The listing builds one solid part. Answer for the finished solid, in the listing's coordinates (mm). A direction names the side the tool comes from. Round coordinates to 2 decimals unless told otherwise and drop trailing zeros. Loops run counter-clockwise (first coordinate to the right, second up) from the corner with the lowest first, then second, coordinate; pieces in that order, holes last. Notation, with made-up numbers: M -33.75,24 L 24.25,24 A21 cw 24.25,36 Z; hole C -18,-35 d5. An arc over 180 degrees is marked long. Put each result on its own line as item: value. Start each with the question number.
(1) Determine the mould class of faces 4 (the face through (54, -2, -72)), 5 (the face through (34.359, -1.726, 79.113)), 6 (the face through (42.922, -1.726, -52.965)) for opening direction Z: released by +Z, released by -Z, zero draft, split by the parting line, or undercut.
(2) Straight lines are drawn through the part: line 1 (Z direction, x = 46, y = -2.2); line 2 (Z direction, x = 73.5, y = -1.1); line 3 (X direction, y = -2.25, z = -44). For each, find the intervals that lie inside material, in ascending order.
(3) Section B-B, the plane y = -2.25 is taken. Count the separate pieces of the cut face and the enclosed holes in it, then the cut area to 3 significant figures.
(4) Section D-D, the plane z = -35 is taken. Determine the outline of the cut face in (x, y), then the cut area to 3 significant figures.
(5) Section C-C, the plane z = 3 is taken. Determine the outline of the cut face in (x, y), then the cut area to 3 significant figures.
(6) Which of the six approach directions +Z, -Z, +X, -X, +Y, -Y give full straight-line access (tool end or side, diameter ignored) to faces 1 (the face through (50.873, -2, -47)), 2 (the face through (60.112, -1.726, 66.981)), 3 (the face through (59.328, -1.726, -3.284))?
(7) Flat-ended cylindrical pins translate along their axes: P1, Ø0.7, axis at y = -2.5, z = -43, coming from the -X side; P2, Ø2, axis at x = 77.5, y = -2, coming from the +Z side; P3, Ø1, axis at y = -1.5, z = -48, coming from the -X side. Find the tip coordinate at first contact, or state that the pin passes through.
(8) Section A-A, the plane x = 45 is taken. Determine the outline of the cut face in (y, z), then the cut area to 3 significant figures.
```python
from build123d import *

# Parameters (mm, degrees)
F1_DEPTH = 3.5
F2_D     = 7.5
F4_DEPTH = 25


with BuildPart() as f1:
    # F0 (on Front) → F1 (new body)
    with BuildSketch(Plane.XZ):
        with BuildLine():
            ThreePointArc((41.4336819508, -79.5), (42.1706374775, -79.4080743718), (42.8624296043, -79.1379310345))
            ThreePointArc((42.8624296043, -79.1379310345), (90, 0), (42.8624296043, 79.1379310345))
            ThreePointArc((42.8624296043, 79.1379310345), (42.1706374775, 79.4080743718), (41.4336819508, 79.5))
            Line((41.4336819508, 79.5), (35.8331652233, 79.5))
            ThreePointArc((35.8331652233, 79.5), (34.3404775581, 79.1022842916), (33.2435667811, 78.0145890229))
            ThreePointArc((33.2435667811, 78.0145890229), (30.1884169541, 62.5971202701), (37.3284684526, 48.5952651142))
            ThreePointArc((37.3284684526, 48.5952651142), (37.696787223, 48.2936203298), (38.1081859652, 48.054038679))
            ThreePointArc((38.1081859652, 48.054038679), (53.4450002112, 35.0932650584), (60.5514057613, 16.3129955125))
            ThreePointArc((60.5514057613, 16.3129955125), (60.556983556, 16.2276326693), (60.5552452702, 16.1421054506))
            Line((60.5552452702, 16.1421054506), (58.0653059802, -23.2613034815))
            ThreePointArc((58.0653059802, -23.2613034815), (53.3089478497, -34.9939813299), (42.4604654753, -41.5200139942))
            ThreePointArc((42.4604654753, -41.5200139942), (41.8979228629, -41.8706217716), (41.6782328608, -42.4960146939))
            Line((41.6782328608, -42.4960146939), (41.6782328608, -43.8381428359))
            ThreePointArc((41.6782328608, -43.8381428359), (41.7451451632, -44.1977917599), (41.9369275579, -44.5093108088))
            ThreePointArc((41.9369275579, -44.5093108088), (44.4656332073, -45.4380618454), (46.6673711793, -43.8858760796))
            ThreePointArc((46.6673711793, -43.8858760796), (47.0897331674, -43.4580841529), (47.6810548772, -43.3497595621))
            Line((47.6810548772, -43.3497595621), (49.9965035646, -43.6386380299))
            ThreePointArc((49.9965035646, -43.6386380299), (50.6223024281, -43.9690543814), (50.8727020195, -44.6309450275))
            Line((50.8727020195, -44.6309450275), (50.8727020195, -49.0738430408))
            ThreePointArc((50.8727020195, -49.0738430408), (50.7018924929, -49.6328091926), (50.2478157018, -50.0008218568))
            Line((50.2478157018, -50.0008218568), (35.3876870019, -56.0141605654))
            ThreePointArc((35.3876870019, -56.0141605654), (34.4991811471, -56.7215784312), (34.1391186959, -57.7987217467))
            ThreePointArc((34.1391186959, -57.7987217467), (33.9649542689, -66.7004891105), (34.0604191652, -75.6034482759))
            ThreePointArc((34.0604191652, -75.6034482759), (35.2674681933, -78.3647681497), (38.0590812482, -79.5))
            Line((38.0590812482, -79.5), (41.4336819508, -79.5))
        make_face()
    extrude(amount=F1_DEPTH)

    # F2 (through all)
    with Locations(Plane(origin=(0, 0, 0), x_dir=(1, 0, 0), z_dir=(0, 1, 0))):
        with Locations((73.0777548589, 16.8713290758), (43.6170464707, 64.6649306593)):
            Hole(F2_D / 2)

    # F3 (on face) → F4 (cut)
    with BuildSketch(Plane.XZ.offset(3.5)):
        with BuildLine():
            Line((76.6596311124, 44.2594586587), (77.9422863406, 45))
            ThreePointArc((77.9422863406, 45), (75.9052301232, 48.3569647512), (73.723683986, 51.6218792716))
            Line((73.723683986, 51.6218792716), (72.305921722, 50.629151447))
            ThreePointArc((72.305921722, 50.629151447), (71.8946904054, 49.9836475804), (72.0603461141, 49.2364229663))
            Line((72.0603461141, 49.2364229663), (75.3404790681, 44.5519076262))
            ThreePointArc((75.3404790681, 44.5519076262), (75.9431914985, 44.1491880554), (76.6596311124, 44.2594586587))
        make_face()
        with BuildLine():
            Line((74.3439292434, -44.5647694037), (73.723683986, -51.6218792716))
            ThreePointArc((73.723683986, -51.6218792716), (75.9052301232, -48.3569647512), (77.9422863406, -45))
            Line((77.9422863406, -45), (75.8400892015, -43.7862959158))
            ThreePointArc((75.8400892015, -43.7862959158), (74.8785169765, -43.7652186868), (74.3439292434, -44.5647694037))
        make_face()
        with BuildLine():
            Line((65.4019169356, -56.7492744962), (63.6396103068, -63.6396103068))
            ThreePointArc((63.6396103068, -63.6396103068), (66.3549603129, -60.8031186854), (68.9439998807, -57.8508848718))
            Line((68.9439998807, -57.8508848718), (67.0135186397, -56.2310187745))
            ThreePointArc((67.0135186397, -56.2310187745), (66.0645928824, -56.0450761197), (65.4019169356, -56.7492744962))
        make_face()
    extrude(amount=-F4_DEPTH, mode=Mode.SUBTRACT)


solid = f1.part
```
Recorded:
1. face 4: released by -Z
1. face 5: released by +Z
1. face 6: undercut
2. line 1: z = -77.36 to -67.56, -61.77 to -51.72, -44.74 to -40.38, 43.05 to 77.36
2. line 2: z = -51.94 to -20.6, -13.15 to 47.18, 51.47 to 51.94
2. line 3: x = 41.69 to 46.61, 50.65 to 74.58, 76.21 to 78.51
3. separate pieces: 1
3. enclosed holes: 2
3. area: 4,490 mm²
4. outline: M 53.3,-3.5 L 82.92,-3.5 L 82.92,0 L 53.3,0 Z
4. area: 104 mm²
5. outline: M 59.72,-3.5 L 89.95,-3.5 L 89.95,0 L 59.72,0 Z
5. area: 106 mm²
6. face 1: +Y, -Y
6. face 2: +Z, +X, +Y, -Y
6. face 3: -X, +Y, -Y
7. P1: stops at x = 41.68
7. P2: stops at z = 45
7. P3: stops at x = 50.87
8. outline: M -3.5,-77.94 L 0,-77.94 L 0,-68.15 L -3.5,-68.15 Z; M -3.5,-61.18 L 0,-61.18 L 0,-52.12 L -3.5,-52.12 Z; M -3.5,-45.32 L 0,-45.32 L 0,-40.77 L -3.5,-40.77 Z; M -3.5,43.84 L 0,43.84 L 0,77.94 L -3.5,77.94 Z
8. area: 201 mm²
